Check sheet for the modelled part. Datum: model origin and axes. Units: mm. A direction names the side the tool comes from. Give positions to 0.01 mm unless a question says otherwise; leave off trailing zeros. Order: outer loops, then holes, each group sorted by start corner. A loop starts at its lowest first (then second) coordinate and runs counter-clockwise, first axis right, second up.
```python
from build123d import *

# Parameters (mm, degrees)
BOSS_EXTRUDE1_DEPTH     = 74
CUT_EXTRUDE1_DEPTH      = 100
SKETCH3_R               = 5
CUT_EXTRUDE2_DEPTH      = 100
BOSS_EXTRUDE2_START     = -3.949924481
BOSS_EXTRUDE2_OUTLINE_R = 30
BOSS_EXTRUDE2_DEPTH     = 10
BOSS_EXTRUDE3_START     = 6.050075519
BOSS_EXTRUDE3_OUTLINE_R = 21
BOSS_EXTRUDE3_DEPTH     = 40
BOSS_EXTRUDE4_START     = 46.050075519
BOSS_EXTRUDE4_OUTLINE_R = 17.5
BOSS_EXTRUDE4_DEPTH     = 105
FILLET1_R               = 1
CUT_EXTRUDE3_START      = -65
CUT_EXTRUDE3_DEPTH      = 65
CUT_EXTRUDE4_START      = -10
CUT_EXTRUDE4_DEPTH      = 10


# Read off the part's stored shape, not the designer's step: Boss-Extrude2, Boss-Extrude3, Boss-Extrude4
with BuildPart() as part:
    # Sketch1 → Boss-Extrude1 (new body)
    with BuildSketch(Plane.XY):
        Polygon((-61.949924481, 30.103941839), (-61.949924481, 20.103941839), (-13.949924481, 20.103941839), (-13.949924481, -35.896058161), (-61.949924481, -35.896058161), (-61.949924481, -45.896058161), (-3.949924481, -45.896058161), (-3.949924481, 30.103941839), align=None)
    extrude(amount=BOSS_EXTRUDE1_DEPTH)

    # Sketch2 → Cut-Extrude1 (cut)
    with BuildSketch(Plane(origin=(0, 30.103941839, 0), x_dir=(1, 0, 0), z_dir=(0, 1, 0))):
        with BuildLine():
            Line((-61.949924481, 0), (-61.949924481, -37))
            ThreePointArc((-61.949924481, -37), (-59.294185522, -28.478308892), (-52.267361901, -22.974136059))
            Line((-52.267361901, -22.974136059), (-3.949924481, 0))
            Line((-3.949924481, 0), (-61.949924481, 0))
        make_face()
        with BuildLine():
            Line((-61.949924481, -74), (-3.949924481, -74))
            Line((-3.949924481, -74), (-54.47214826, -49.97752478))
            ThreePointArc((-54.47214826, -49.97752478), (-59.946719407, -44.488879866), (-61.949924481, -37))
            Line((-61.949924481, -37), (-61.949924481, -74))
        make_face()
    extrude(amount=-CUT_EXTRUDE1_DEPTH, mode=Mode.SUBTRACT)

    # Sketch3 → Cut-Extrude2 (cut)
    with BuildSketch(Plane(origin=(0, 30.103941839, 0), x_dir=(1, 0, 0), z_dir=(0, 1, 0))):
        with Locations(Location((-46.949924481, -37, 0), (0, 0, 180))):
            Circle(SKETCH3_R)
    extrude(amount=-CUT_EXTRUDE2_DEPTH, mode=Mode.SUBTRACT)

    # Boss-Extrude2 outline → Boss-Extrude2 (add)
    with BuildSketch(Plane.YZ.offset(BOSS_EXTRUDE2_START)):
        with Locations((-7.896058161, 37)):
            Circle(BOSS_EXTRUDE2_OUTLINE_R)
    extrude(amount=BOSS_EXTRUDE2_DEPTH)

    # Boss-Extrude3 outline → Boss-Extrude3 (add)
    with BuildSketch(Plane.YZ.offset(BOSS_EXTRUDE3_START)):
        with Locations((-7.896058161, 37)):
            Circle(BOSS_EXTRUDE3_OUTLINE_R)
    extrude(amount=BOSS_EXTRUDE3_DEPTH)

    # Boss-Extrude4 outline → Boss-Extrude4 (add)
    with BuildSketch(Plane.YZ.offset(BOSS_EXTRUDE4_START)):
        with Locations((-7.896058161, 37)):
            Circle(BOSS_EXTRUDE4_OUTLINE_R)
    extrude(amount=BOSS_EXTRUDE4_DEPTH)

    # Fillet1
    fillet1_edges = [part.edges().sort_by_distance(p)[0] for p in [
        (151.050075519, -25.396058161, 37),
    ]]
    fillet(fillet1_edges, radius=FILLET1_R)

    # Sketch4 → Cut-Extrude3 (cut)
    with BuildSketch(Plane(origin=(151.050075519, 0, 0), x_dir=(0, 0, -1), z_dir=(1, 0, 0)).offset(CUT_EXTRUDE3_START)):
        with BuildLine():
            Line((-52.811388301, -0.396058161), (-21.188611699, -0.396058161))
            ThreePointArc((-21.188611699, -0.396058161), (-37, 9.603941839), (-52.811388301, -0.396058161))
        make_face()
    extrude(amount=CUT_EXTRUDE3_DEPTH, mode=Mode.SUBTRACT)

    # Sketch5 → Cut-Extrude4 (cut)
    with BuildSketch(Plane(origin=(6.050075519, 0, 0), x_dir=(0, 0, -1), z_dir=(1, 0, 0)).offset(CUT_EXTRUDE4_START)):
        with BuildLine():
            Line((-22.033370453, 18.103941839), (-51.966629547, 18.103941839))
            ThreePointArc((-51.966629547, 18.103941839), (-37, 22.103941839), (-22.033370453, 18.103941839))
        make_face()
        with BuildLine():
            Line((-51.966629547, -33.896058161), (-22.033370453, -33.896058161))
            ThreePointArc((-22.033370453, -33.896058161), (-37, -37.896058161), (-51.966629547, -33.896058161))
        make_face()
    extrude(amount=CUT_EXTRUDE4_DEPTH, mode=Mode.SUBTRACT)


solid = part.part
```
(1) Gauge pin test, flat ends, axial feed: pin 1 Ø6 at (y, z) = (4.5, 56.5) entering from -X; pin 2 Ø12 at (x, z) = (27.5, 49) entering from -Y; pin 3 Ø8 at (x, z) = (2.5, 39) entering from +Y. Record the tip position at first contact, or that the pin passes through.
Response values:
pin 1: stops at x = -13.95
pin 2: stops at y = -28.02
pin 3: stops at y = 18.1
(2) Release check for a two-part mould opening along X. For faces 1 (the face through (-49.638, -40.826, 41.216)), 2 (the face through (0.98, -7.456, 66.997)), 3 (the face through (-12.017, -7.364, 70.164)) record: released by +X, released by -X, zero draft, split by the parting line, or undercut.
Response values:
face 1: undercut
face 2: zero draft
face 3: released by -X
(3) Cross-section at B-B on z = 63.5. Enter the section's corners in (x, y).
Response values:
outline: (-26.03, -45.9) - (-3.95, -45.9) - (-3.95, -21.96) - (6.05, -21.96) - (6.05, 6.17) - (-3.95, 6.17) - (-3.95, 30.1) - (-26.03, 30.1) - (-26.03, 20.1) - (-13.95, 20.1) - (-13.95, -35.9) - (-26.03, -35.9) - close
(4) Cross-section at D-D on x = 134. Enter the section's corners in (y, z).
Response values:
outline: (-0.4, 21.19) - (-0.4, 52.81) arc R17.5 ccw (long way) to start
(5) Set-up check for faces 4 (the face through (46.05, -16, 53)), 5 (the face through (1, -33.896, 37)), 6 (the face through (86.05, 4, 37)), 7 (the face through (-13.95, -8, 37)), 8 (the face through (1, -8, 7)): record each of +Z, -Z, +X, -X, +Y, -Y from which the full face is reachable in a straight line by a thin tool's end or side.
Response values:
face 4: +X
face 5: +Z, -Z, +X, -Y
face 6: +Z, -Z, +X, +Y
face 7: +Z, -Z, -X
face 8: -Z, +X
(6) Material ranges on L1, parallel to Y at x = -15, z = 56; L2, parallel to X at y = 14, z = 47; L3, parallel to X at y = 5.5, z = 67.5, recorded low to high.
Response values:
L1: y = -45.9 to -35.9, 20.1 to 30.1
L2: x = -13.95 to 6.05
L3: x = -13.95 to -3.95
(7) Cross-section at A-A on y = 16. Enter the section's corners in (x, z).
Response values:
outline: (-13.95, 4.75) - (-3.95, 0) - (-3.95, 18.86) - (6.05, 18.86) - (6.05, 55.14) - (-3.95, 55.14) - (-3.95, 74) - (-13.95, 69.25) - close
(8) Cross-section at C-C on x = 12.5. Enter the section's corners in (y, z), then the cut area to 3 significant figures.
Response values:
outline: circle Ø42 at (-7.9, 37)
area: 1,390 mm2
